Here's the drawing with two shaded views (mm, measured from the low corner). I have some questions. Coordinates: 2 decimals unless noted, no trailing zeros. Write each loop counter-clockwise with the first axis right and the second up, starting at its lowest first coordinate (ties: lowest second). Pieces come first, ordered by that corner, then holes. Notation, with made-up numbers: M 9.25,25 L 33.25,25 A16 ccw 33.25,55 Z; hole C 23,73.5 d2. An arc over 180 degrees is marked long. Answer as CSV lines item,"result". Start each with the question number.
Item 1: If I drill on line 1 along Z through (x, y) = (110, 0.8); line 2 along Z through (x, y) = (10, 0.8); line 3 along X through (y, z) = (1.65, 26), over which ranges is the centre line in solid material (lowest first)? Write a range as [from, to].
Item 2: Suppose I cut it at A-A, the plane z = 25. Write out the boundary of the cut face in (x, y).
Item 3: Suppose I cut it at B-B, the plane x = 210. Write out the boundary of the cut face in (y, z), and give its area (3 significant figures).
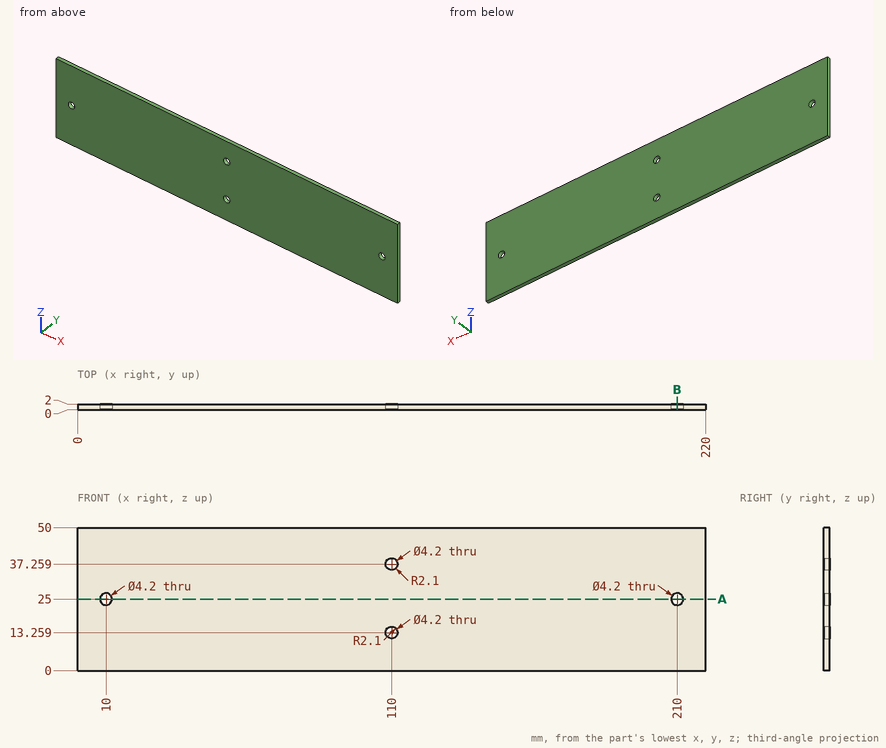
Ans:
1,line 1,"z = [0, 11.16], [15.36, 35.16], [39.36, 50]"
1,line 2,"z = [0, 22.9], [27.1, 50]"
1,line 3,"x = [0, 8.15], [11.85, 208.15], [211.85, 220]"
2,outline,"M 0,0 L 7.9,0 L 7.9,2 L 0,2 Z; M 12.1,0 L 207.9,0 L 207.9,2 L 12.1,2 Z; M 212.1,0 L 220,0 L 220,2 L 212.1,2 Z"
3,outline,"M 0,0 L 2,0 L 2,22.9 L 0,22.9 Z; M 0,27.1 L 2,27.1 L 2,50 L 0,50 Z"
3,area,"91.6 mm^2"
